Autodesk Inventor part; units mm, degrees
ref_plane "YZ Plane" through (0, 0, 0) normal (1, 0, 0) x (0, 1, 0)
ref_plane "XZ Plane" through (0, 0, 0) normal (0, 1, 0) x (-1, 0, 0)
ref_plane "XY Plane" through (0, 0, 0) normal (0, 0, 1) x (1, 0, 0)
sketch "スケッチ1" plane through (0, 0, 0) normal (0, 0, 1) x (1, 0, 0)
  line L0 (-11.5, 17) -> (11.5, 17)
  line L1 (11.5, 17) -> (11.5, 0)
  line L2 (11.5, 0) -> (-11.5, 0)
  line L3 (-11.5, 0) -> (-11.5, 17)
  point P0 (0, 0)
  point P1 (0, 0)
  dimension "d0" = 23
  dimension "d1" = 17
extrude "押し出し1" add sketch "スケッチ1" along normal blind 6
sketch "スケッチ5" plane through (0, 0, 0) normal (0, 0, -1) x (-1, 0, 0)
  line L0 (-11.5, 0) -> (11.5, 0)
  point P0 (0, 0)
  point P1 (-4, 5)
  point P2 (4, 5)
  dimension "d13" = 4
  dimension "d14" = 4
  dimension "d15" = 5
hole "穴1" at (4, 5, 0) at (-4, 5, 0) direction (0, 0, 1) diameter 4.5 end through all counterbore diameter 8 counterbore depth 4.5
sketch "スケッチ6" plane through (0, 0, 0) normal (0, 0, -1) x (-1, 0, 0)
  circle A0 centre (4, 5) radius 4
  circle A1 centre (-4, 5) radius 4
  line L0 (-4, 9) -> (4, 9)
  line L1 (-3.6249, 1.0176) -> (3.9907, 1)
  point P0 (0, 5)
  point P1 (0, 0)
extrude "押し出し5" cut sketch "スケッチ6" against normal up to surface (4.5 mm away) contours A0 A1 L0 | L1 A1 A0
sketch "スケッチ9" plane through (0, 0, 6) normal (0, 0, 1) x (1, 0, 0)
  line L0 (11.5, 17) -> (11.5, 0)
  line L1 (-11.5, 17) -> (11.5, 17)
  line L2 (-11.5, 0) -> (-11.5, 17)
  line L3 (11.5, 0) -> (-11.5, 0)
  line L4 (-11.5, 10) -> (11.5, 10)
  point P0 (0, 0)
  dimension "d32" = 10
extrude "押し出し8" add sketch "スケッチ9" along normal blind 4 contours L0 L4 L2 L1
properties part number "05" material "SUS303"
Design review of the part built by this model. Coordinates are the model's own, in mm. A direction names the side the tool comes from. Round coordinates to 2 decimals unless told otherwise and drop trailing zeros. Write each loop counter-clockwise with the first axis right and the second up, starting at its lowest first coordinate (ties: lowest second). Pieces come first, ordered by that corner, then holes. Notation, with made-up numbers: (37, -19) -> (66, -19) arc R17 ccw to (66, -8) -> close; hole circle Ø5 at (45.5, 32). An arc over 180 degrees is marked (long way). Answer in a Markdown table with one row per item.
Q1. Take a section at D-D, the plane z = 2.75. State the section outline as (x, y) points, then the cut area to 3 significant figures.
The answers:
| item | result |
|---|---|
| outline | (-11.5, 0) -> (11.5, 0) -> (11.5, 17) -> (-11.5, 17) -> close; hole (-4, 9) arc R4 ccw to (-3.99, 1) -> (3.62, 1.02) arc R4 ccw (long way) to (4, 9) -> close |
| area | 277 mm² |
Q2. Take a section at A-A, the plane y = 5. State the section outline as (x, z) points.
The answers:
| item | result |
|---|---|
| outline | (-11.5, 0) -> (-8, 0) -> (-8, 4.5) -> (-6.25, 4.5) -> (-6.25, 6) -> (-11.5, 6) -> close; (-1.75, 4.5) -> (1.75, 4.5) -> (1.75, 6) -> (-1.75, 6) -> close; (6.25, 4.5) -> (8, 4.5) -> (8, 0) -> (11.5, 0) -> (11.5, 6) -> (6.25, 6) -> close |
Q3. For faces 5 (the face through (0, 9, 2)), 6 (the face through (0, 0, 3)), 7 (the face through (0, 5, 6)), list the 3-axis set-ups (+Z, -Z, +X, -X, +Y, -Y) from which the entire face can be reached by the end or side of a thin tool; tool diameter is ignored.
The answers:
| item | result |
|---|---|
| face 5 | -Z |
| face 6 | +Z, -Z, +X, -X, -Y |
| face 7 | +Z, +X, -X, -Y |
Q4. Take a section at C-C, the plane x = -5. State the section outline as (y, z) points, then the cut area to 3 significant figures.
The answers:
| item | result |
|---|---|
| outline | (0, 0) -> (1.13, 0) -> (1.13, 4.5) -> (2.98, 4.5) -> (2.98, 6) -> (0, 6) -> close; (7.02, 4.5) -> (8.87, 4.5) -> (8.87, 0) -> (17, 0) -> (17, 10) -> (10, 10) -> (10, 6) -> (7.02, 6) -> close |
| area | 89.1 mm² |
Q5. To check wall thickness, follow L1, parallel to Y at x = -4, z = 5.3; L2, parallel to X at y = 5, z = 5.5; L3, parallel to Y at x = -1, z = 1. State the ranges of each line that lie inside material, in increasing order. Write a range as [from, to].
The answers:
| item | result |
|---|---|
| L1 | [0, 2.75], [7.25, 17] |
| L2 | [-11.5, -6.25], [-1.75, 1.75], [6.25, 11.5] |
| L3 | [0, 1.01], [9, 17] |
Q6. Clearance check with flat-ended pins moving along their axes: pin 1 Ø8 at (x, y) = (5, 3) entering from -Z; pin 2 Ø2.5 at (x, y) = (-4, 5) entering from +Z; pin 3 Ø6 at (x, y) = (-2.5, 5.5) entering from -Z; pin 4 Ø1.2 at (x, z) = (0, 8) entering from -Y. State where each tip first meets the part, or that it passes through.
The answers:
| item | result |
|---|---|
| pin 1 | z = 0 |
| pin 2 | through |
| pin 3 | z = 4.5 |
| pin 4 | y = 10 |
Q7. Take a section at B-B, the plane z = 5. State the section outline as (x, y) points, then the cut area to 3 significant figures.
The answers:
| item | result |
|---|---|
| outline | (-11.5, 0) -> (11.5, 0) -> (11.5, 17) -> (-11.5, 17) -> close; hole circle Ø4.5 at (-4, 5); hole circle Ø4.5 at (4, 5) |
| area | 359 mm² |
Q8. Draft analysis for pull direction Y (two halves, no side actions). For faces 1 (the face through (-11.5, 10, 4)), 2 (the face through (-8, 5, 2)), 3 (the face through (0, 10, 8)), 4 (the face through (8, 5, 2)), state which applies: +Y half, -Y half, draft (parallel to the pull), parting line (faces both ways), or undercut.
The answers:
| item | result |
|---|---|
| face 1 | draft |
| face 2 | undercut |
| face 3 | -Y half |
| face 4 | undercut |
